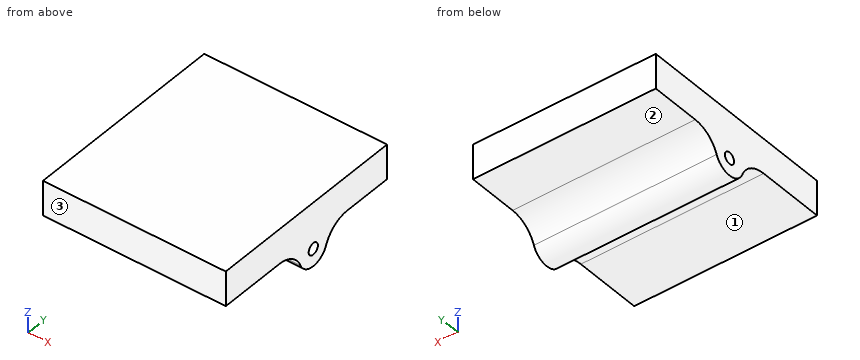
from build123d import *

# Parameters (mm, degrees)
F0_W     = 31.5
F0_H     = 35
F1_DEPTH = 6
F3_DEPTH = 31.5
F4_R     = 5


# Not quite as in the source:
# - a feature of the source that left no trace in its solid (it failed there, or was rolled back) is left out


with BuildPart() as f1:
    # F0 (on Top) → F1 (new body)
    with BuildSketch(Plane.XY):
        with Locations((15.75, 17.5)):
            Rectangle(F0_W, F0_H)
    extrude(amount=F1_DEPTH)

    # F2 (on face) → F3 (join, through all)
    with BuildSketch(Plane.YZ.offset(31.5)):
        with BuildLine():
            Line((22, -2), (22, 0))
            Line((22, 0), (16, 0))
            Line((16, 0), (16, -2))
            Line((16, -2), (18, -2))
            ThreePointArc((18, -2), (19, -1), (20, -2))
            Line((20, -2), (22, -2))
        make_face()
        with BuildLine():
            ThreePointArc((16, -2), (19, -5), (22, -2))
            Line((22, -2), (20, -2))
            ThreePointArc((20, -2), (19, -3), (18, -2))
            Line((18, -2), (16, -2))
        make_face()
    extrude(amount=-F3_DEPTH)

    # F4
    f4_edges = [f1.edges().sort_by_distance(p)[0] for p in [
        (15.75, 22, 0),
        (15.75, 16, 0),
    ]]
    fillet(f4_edges, radius=F4_R)


solid = f1.part
CAD build for the part. Positions are in the model's coordinates, mm. Face numbers are marked on the shaded views. A direction names the side the tool comes from. Round coordinates to 2 decimals unless told otherwise and drop trailing zeros. Order: outer loops, then holes, each group sorted by start corner. A loop starts at its lowest first (then second) coordinate and runs counter-clockwise, first axis right, second up. Notation, with made-up numbers: (52, 56.25) -> (96, 56.25) arc R36 cw to (96, 90.25) -> close; hole circle Ø7 at (47.25, 42.25). An arc over 180 degrees is marked (long way). Write item = value, one per line. Start each with the question number.
(1) Cut at B-B, the plane y = 8. List the corners of the cut face in (x, z).
(2) Probe line 1 (Z direction, x = 24.5, y = 19); line 2 (Y direction, x = 16, z = -2); line 3 (Y direction, x = 28, z = -1.5). List the from-to ranges inside material, lowest first. Write a range as [from, to].
(3) Cut at A-A, the plane y = 19. List the corners of the cut face in (x, z), then the cut area to 4 significant figures.
(4) Pin check, flat tip, straight feed: P1, Ø12.5, axis at x = 21, y = 6, coming from the -Z side. Stop position of the tip, or through.
(5) Which spindle directions (+Z, -Z, +X, -X, +Y, -Y) get a long thin tool onto all of the face, cutting with end or side? Do the marked faces 1, 2 and 3. Say none if no direction does.
Model answer:
q1.outline = (0, 0) -> (31.5, 0) -> (31.5, 6) -> (0, 6) -> close
q2.line_1 = [-5, -3], [-1, 6]
q2.line_2 = [15.58, 18], [20, 22.42]
q2.line_3 = [15.15, 18.13], [19.87, 22.85]
q3.outline = (0, -5) -> (31.5, -5) -> (31.5, -3) -> (0, -3) -> close; (0, -1) -> (31.5, -1) -> (31.5, 6) -> (0, 6) -> close
q3.area = 283.5 mm2
q4.P1 = -0.04
q5.face_1 = -Z, +X, -X, -Y
q5.face_2 = -Z, +X, -X, +Y
q5.face_3 = +Z, -Z, +X, -X, -Y
